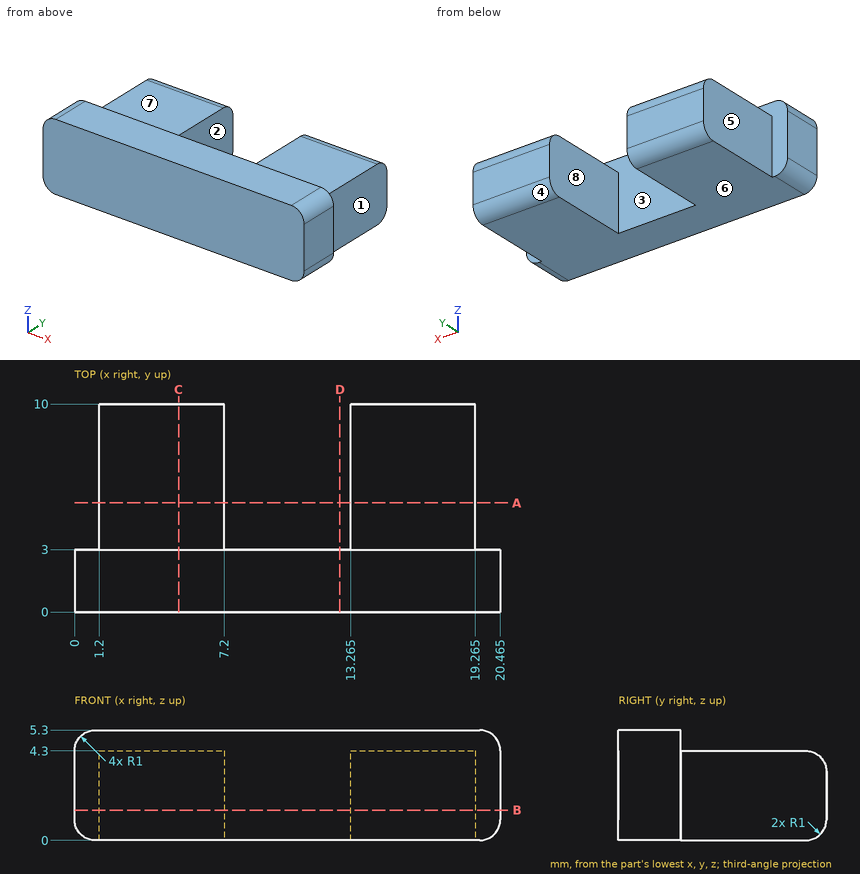
Check sheet for the drawn part. Datum: minimum x, y, z corner. Units: mm. A direction names the side the tool comes from. Round coordinates to 2 decimals unless told otherwise and drop trailing zeros. Loops run counter-clockwise (first coordinate to the right, second up) from the corner with the lowest first, then second, coordinate; pieces in that order, holes last. Notation, with made-up numbers: (-4.75, -28.75) - (35.25, -28.75) arc R32 cw to (35.25, 2.25) - close; hole circle Ø3 at (-3, -24). An arc over 180 degrees is marked (long way). Write item = value, one per line. Start each with the question number.
1. Set-up check for the marked faces 5, 6, 7 and 8: record each of +Z, -Z, +X, -X, +Y, -Y from which the full face is reachable in a straight line by a thin tool's end or side.
2. Section check A-A on y = 5.25. Enter the section's corners in (x, z) (3 decimals).
3. Mould release check, pull along X, two halves, no side actions. Record for the marked faces 1, 2, 3 and 4: released by +X, released by -X, zero draft, split by the parting line, or undercut.
4. Depth check by flat-ended pin: pin 1 (5 mm diameter, centred on x = 6.5, y = 6, fed in from +Z); pin 2 (1.3 mm diameter, centred on y = 6, z = 2.5, fed in from -X); pin 3 (1.3 mm diameter, centred on y = 6, z = 2, fed in from +X) (3 decimals). Enter the tip coordinate at first touch or a pass-through.
5. Section check C-C on x = 5. Enter the section's corners in (y, z).
6. Section check B-B on z = 1.45. Enter the section's corners in (x, y) (3 decimals), then the cut area to 3 significant figures.
7. Thickness scan on line 1 (X direction, y = 9.25, z = 1.3) (3 decimals); line 2 (Y direction, x = 10.5, z = 2.05); line 3 (Z direction, x = 3.75, y = 8.25). Record the ranges inside material, lowest first.
8. Section check D-D on x = 12.75. Enter the section's corners in (y, z).
Working result:
q1.face_5 = +Z, -Z, -X, +Y
q1.face_6 = -Z, +X, -X, +Y, -Y
q1.face_7 = +Z, +X, -X, +Y
q1.face_8 = +Z, -Z, +Y
q2.outline = (1.2, 0) - (7.2, 0) - (7.2, 4.3) - (1.2, 4.3) - close; (13.265, 0) - (19.265, 0) - (19.265, 4.3) - (13.265, 4.3) - close
q3.face_1 = released by +X
q3.face_2 = undercut
q3.face_3 = undercut
q3.face_4 = zero draft
q4.pin_1 = 4.3
q4.pin_2 = 1.2
q4.pin_3 = 19.265
q5.outline = (0, 0) - (9, 0) arc R1 ccw to (10, 1) - (10, 3.3) arc R1 ccw to (9, 4.3) - (3, 4.3) - (3, 5.3) - (0, 5.3) - close
q6.outline = (0, 0) - (20.465, 0) - (20.465, 3) - (19.265, 3) - (19.265, 10) - (13.265, 10) - (13.265, 3) - (7.2, 3) - (7.2, 10) - (1.2, 10) - (1.2, 3) - (0, 3) - close
q6.area = 145 mm^2
q7.line_1 = 1.2 to 7.2, 13.265 to 19.265
q7.line_2 = 0 to 3
q7.line_3 = 0 to 4.3
q8.outline = (0, 0) - (3, 0) - (3, 5.3) - (0, 5.3) - close
